Part model, mm, in its own coordinate system. A direction names the side the tool comes from. Round coordinates to 2 decimals unless told otherwise and drop trailing zeros. Write each loop counter-clockwise with the first axis right and the second up, starting at its lowest first coordinate (ties: lowest second). Pieces come first, ordered by that corner, then holes. Notation, with made-up numbers: (-7, -6) -> (20, -6) arc R31 ccw to (20, 32) -> close; hole circle Ø1 at (23, -11). An arc over 180 degrees is marked (long way). Return JSON: item names as keys, results as strings. Group by question number.
(1) Saw through at A-A (z = 1.4). List the corners of the cut face in (x, y), plus the area to 3 significant figures.
(2) Saw through at B-B (x = -3). List the corners of the cut face in (y, z).
(3) Tool access for faces 4 (the cylindrical face through (34.43, 9.4, 2.03)), 5 (the flat face through (-6, -0.1, 2)): list every direction of +Z, -Z, +X, -X, +Y, -Y with a clear straight run to the whole face (end or side of a thin tool).
(4) Drill centre lines: L1, parallel to Y at x = 0.3, z = 2.3; L2, parallel to X at y = 6.3, z = 1.9; L3, parallel to Y at x = 22, z = 1.05. Where is each one in solid material? Low to high. Write a range as from..to.
(5) Mould opens along X. For faces 1 (the cylindrical face through (-46.4, 9.43, 2.03)), 2 (the flat face through (0.1, 3, 2)), 3 (the flat face through (-5, 10, 2)) say: +X half, -X half, draft (parallel to the pull), parting line (faces both ways), or undercut.
(6) Saw through at C-C (x = 22). List the corners of the cut face in (y, z), plus the area to 3 significant figures.
Autodesk Inventor part; units mm, degrees
ref_plane "YZ Plane" through (0, 0, 0) normal (1, 0, 0) x (0, 1, 0)
ref_plane "XZ Plane" through (0, 0, 0) normal (0, 1, 0) x (-1, 0, 0)
ref_plane "XY Plane" through (0, 0, 0) normal (0, 0, 1) x (1, 0, 0)
ref_plane "작업 평면1" through (0, 0, 0) normal (0, 0, 1) x (1, 0, 0)
sketch "스케치1" plane through (0, 0, 0) normal (0, 0, 1) x (1, 0, 0)
  line L0 (-12, 0) -> (0, 0)
  line L1 (0, 0) -> (0, 6)
  line L2 (-12, 6) -> (0, 6)
  line L3 (-12, 0) -> (-12, 6)
  line L4 (0.3, -0.3) -> (-12.3, -0.3)
  line L5 (-12.3, -0.3) -> (-12.3, 6.3)
  line L6 (-12.3, 6.3) -> (0.3, 6.3)
  line L7 (0.3, 6.3) -> (0.3, -0.3)
  line L8 (4, -4) -> (-16, -4)
  line L9 (-16, -4) -> (-16, 10)
  line L10 (-16, 10) -> (4, 10)
  line L11 (4, 10) -> (4, -4)
  line L12 (1, 6) -> (1, 0)
  line L13 (1, 0) -> (31, 0)
  line L14 (31, 0) -> (31, 6)
  line L15 (1, 6) -> (31, 6)
  circle A0 centre (22, 3.1) radius 1.35
  line L16 (-13, 0) -> (-13, 6)
  line L17 (-43, 6) -> (-13, 6)
  line L18 (-43, 0) -> (-43, 6)
  line L19 (-43, 0) -> (-13, 0)
  circle A1 centre (-34, 3.1) radius 1.35
  line L20 (31, 0) -> (-43, 0)
  line L21 (-43, 0) -> (-43, 6)
  line L22 (-43, 6) -> (31, 6)
  line L23 (31, 6) -> (31, 0)
  line L24 (-47, -4) -> (35, -4)
  line L25 (35, -4) -> (35, 10)
  line L26 (35, 10) -> (-47, 10)
  line L27 (-47, 10) -> (-47, -4)
  circle A2 centre (0.3, 6.3) radius 1.05
  circle A3 centre (0.3, -0.3) radius 1.05
  circle A4 centre (-12.3, -0.3) radius 1.05
  circle A5 centre (-12.3, 6.3) radius 1.05
  point P0 (0.3, 5.25)
  point P1 (0.3, 0.75)
  point P2 (-0.75, -0.3)
  point P3 (-11.25, -0.3)
  point P4 (-12.3, 0.75)
  point P5 (-12.3, 5.25)
  point P6 (-11.25, 6.3)
  point P7 (-0.75, 6.3)
  dimension "d0" = 0.3
  dimension "d1" = 4
  dimension "d4" = 2.1
  dimension "d5" = 2.1
  dimension "d6" = 2.1
  dimension "d7" = 2.1
extrude "돌출1" add sketch "스케치1" along normal blind 4 contours L4 A3 L13 L11 L8 L9 L19 A4 | A4 L16 A5 L5 | L19 L9 L17 A5 L16 A4 | L7 A2 L12 A3 | L19 L18 L17 L9 | L9 L24 L27 L26 L17 L18 L19 | A5 L17 L9 L10 L11 L15 A2 L6 | L12 A2 L15 L11 L13 A3 | L13 L14 L15 L11 L26 L25 L24 | L11 L15 L14 L13
sketch "스케치2" plane through (0, 0, 4) normal (0, 0, 1) x (1, 0, 0)
  line L0 (-13, 6) -> (-13, 0)
  line L1 (-42, 0) -> (-13, 0)
  line L2 (-42, 6) -> (-42, 0)
  line L3 (-42, 6) -> (-13, 6)
  circle A0 centre (-17.05, 3) radius 1.35
  point P0 (0, 0)
extrude "돌출2" cut sketch "스케치2" against normal through all contours A0
fillet "모깎기1" radius 2 4 edges at (35, 10, 2) (35, -4, 2) (-47, 10, 2) (-47, -4, 2)
sketch "스케치3" plane through (0, 0, 4) normal (0, 0, 1) x (1, 0, 0)
  circle A0 centre (-17.05, 3) radius 1.35
  arc A1 (-47, -2) -> (-45, -4) centre (-45, -2) ccw
  line L0 (-45, -4) -> (33, -4)
  arc A2 (33, -4) -> (35, -2) centre (33, -2) ccw
  line L1 (35, -2) -> (35, 8)
  arc A3 (35, 8) -> (33, 10) centre (33, 8) ccw
  line L2 (33, 10) -> (-45, 10)
  arc A4 (-45, 10) -> (-47, 8) centre (-45, 8) ccw
  line L3 (-47, 8) -> (-47, -2)
  circle A5 centre (22, 3.1) radius 1.35
  circle A6 centre (-34, 3.1) radius 1.35
  arc A7 (0.3, 5.25) -> (-0.75, 6.3) centre (0.3, 6.3) ccw
  line L4 (0.3, 5.25) -> (0.3, 0.75)
  arc A8 (-0.75, -0.3) -> (0.3, 0.75) centre (0.3, -0.3) ccw
  line L5 (-0.75, -0.3) -> (-11.25, -0.3)
  arc A9 (-12.3, 0.75) -> (-11.25, -0.3) centre (-12.3, -0.3) ccw
  line L6 (-12.3, 0.75) -> (-12.3, 5.25)
  arc A10 (-11.25, 6.3) -> (-12.3, 5.25) centre (-12.3, 6.3) ccw
  line L7 (-11.25, 6.3) -> (-0.75, 6.3)
  line L8 (0.1, 0.5261) -> (0.1, 5.4739)
  arc A11 (0.1, 5.4739) -> (-0.5261, 6.1) centre (0.3, 6.3) ccw
  line L9 (-0.5261, 6.1) -> (-11.4739, 6.1)
  arc A12 (-11.4739, 6.1) -> (-12.1, 5.4739) centre (-12.3, 6.3) ccw
  line L10 (-12.1, 5.4739) -> (-12.1, 0.5261)
  arc A13 (-12.1, 0.5261) -> (-11.4739, -0.1) centre (-12.3, -0.3) ccw
  line L11 (-11.4739, -0.1) -> (-0.5261, -0.1)
  arc A14 (-0.5261, -0.1) -> (0.1, 0.5261) centre (0.3, -0.3) ccw
  point P0 (0, 0)
  dimension "d11" = 0.2
extrude "돌출3" add sketch "스케치3" against normal up to surface (4 mm away) contours L4 A8 L5 A9 L6 A10 L7 A7
properties part number "zig9"
Computed values:
{
 "1": {"outline": "(-47, -2) arc R2 ccw to (-45, -4) -> (33, -4) arc R2 ccw to (35, -2) -> (35, 8) arc R2 ccw to (33, 10) -> (-45, 10) arc R2 ccw to (-47, 8) -> close; hole circle Ø2.7 at (-34, 3.1); hole circle Ø2.7 at (-17.05, 3); hole (-12.1, 0.53) arc R0.85 ccw (long way) to (-11.47, -0.1) -> (-0.53, -0.1) arc R0.85 ccw (long way) to (0.1, 0.53) -> (0.1, 5.47) arc R0.85 ccw (long way) to (-0.53, 6.1) -> (-11.47, 6.1) arc R0.85 ccw (long way) to (-12.1, 5.47) -> close; hole circle Ø2.7 at (22, 3.1)", "area": "1,040 mm2"},
 "2": {"outline": "(-4, 0) -> (-0.1, 0) -> (-0.1, 4) -> (-4, 4) -> close; (6.1, 0) -> (10, 0) -> (10, 4) -> (6.1, 4) -> close"},
 "3": {"face 4": "+Z, -Z, +X, +Y", "face 5": "+Z, -Z"},
 "4": {"L1": "-4..-1.15, 0.55..5.45, 7.15..10", "L2": "-47..-13.15, -11.45..-0.55, 1.15..35", "L3": "-4..1.75, 4.45..10"},
 "5": {"face 1": "-X half", "face 2": "undercut", "face 3": "draft"},
 "6": {"outline": "(-4, 0) -> (1.75, 0) -> (1.75, 4) -> (-4, 4) -> close; (4.45, 0) -> (10, 0) -> (10, 4) -> (4.45, 4) -> close", "area": "45.2 mm2"}
}
